Design review of the part built by this model. Coordinates are the model's own, in mm. A direction names the side the tool comes from. Coordinates: 2 decimals unless noted, no trailing zeros. Loops run counter-clockwise (first coordinate to the right, second up) from the corner with the lowest first, then second, coordinate; pieces in that order, holes last. Notation, with made-up numbers: (27.5, 87.25) -> (77.5, 87.25) arc R20 ccw to (77.5, 113.25) -> close; hole circle Ø7 at (-17, 65.5). An arc over 180 degrees is marked (long way). Answer in a Markdown table with one row per item.
Autodesk Fusion 360 part; units mm, degrees
sketch "Sketch1" plane through (0, 0, 0) normal (0, 1, 0) x (1, 0, 0)
  circle A0 centre (0, 0) radius 61
  dimension "d2" = 122
extrude "Extrude1" add sketch "Sketch1" along normal blind 5
sketch "Sketch3" plane through (0, 5, 0) normal (0, 1, 0) x (-1, 0, 0)
  circle A0 centre (0, 0) radius 61
  circle A1 centre (0, 0) radius 61
  circle A2 centre (0, 0) radius 57.25
  dimension "d5" = 114.5
extrude "Extrude2" add sketch "Sketch3" along normal blind 50
sketch "Sketch4" plane through (0, 5, 0) normal (0, 1, 0) x (-1, 0, 0)
  circle A0 centre (0, 0) radius 57.25
  circle A1 centre (0, 0) radius 45
  dimension "d8" = 90
extrude "Extrude3" cut sketch "Sketch4" against normal blind 55 contours A1
(1) To check wall thickness, follow probe 1 along Z at (x, y) = (0, 37); probe 2 along Z at (x, y) = (0, 1). State the ranges of each line that lie inside material, in increasing order.
Evaluation:
| item | result |
|---|---|
| probe 1 | z = -61 to -57.25, 57.25 to 61 |
| probe 2 | z = -61 to -45, 45 to 61 |
(2) Take a section at A-A on z = 29. Give the boundary of the cut face in (x, y), and give its area (3 significant figures).
Evaluation:
| item | result |
|---|---|
| outline | (-53.67, 0) -> (-34.41, 0) -> (-34.41, 5) -> (-49.36, 5) -> (-49.36, 55) -> (-53.67, 55) -> close; (34.41, 0) -> (53.67, 0) -> (53.67, 55) -> (49.36, 55) -> (49.36, 5) -> (34.41, 5) -> close |
| area | 623 mm² |
(3) Tool access review of faces 5 (the flat face through (-5, 0, 45)), 6 (the flat face through (25, 5, 38)): name each direction out of +Z, -Z, +X, -X, +Y, -Y from which nothing blocks a thin tool from reaching the whole face with its end or side.
Evaluation:
| item | result |
|---|---|
| face 5 | +Z, -Z, +X, -X, -Y |
| face 6 | +Y |
(4) Take a section at D-D on z = 50. Give the boundary of the cut face in (x, y), and give its area (3 significant figures).
Evaluation:
| item | result |
|---|---|
| outline | (-34.94, 0) -> (34.94, 0) -> (34.94, 55) -> (27.88, 55) -> (27.88, 5) -> (-27.88, 5) -> (-27.88, 55) -> (-34.94, 55) -> close |
| area | 1,060 mm² |
(5) For pin 1 (5 mm diameter, centred on y = 32, z = 36, fed in from +X); pin 2 (12 mm diameter, centred on y = 22, z = 34.5, fed in from +X); pin 3 (1.5 mm diameter, centred on x = -37, y = 12, fed in from +Z), all flat-tipped, find the tip position at first contact; note any pin that passes through.
Evaluation:
| item | result |
|---|---|
| pin 1 | stops at x = 50.98 |
| pin 2 | stops at x = 53.93 |
| pin 3 | stops at z = 49.06 |
(6) Take a section at C-C on y = 15. Give the boundary of the cut face in (x, z).
Evaluation:
| item | result |
|---|---|
| outline | circle Ø122 at (0, 0); hole circle Ø114.5 at (0, 0) |
(7) Draft analysis for pull direction Z (two halves, no side actions). For faces 1 (the cylindrical face through (12.41, 29.65, 55.89)), 2 (the flat face through (-18, 55, 55)), 3 (the cylindrical face through (-4.021, 27.115, -60.867)), 4 (the cylindrical face through (-20.765, 2.535, -39.923)), state which applies: pulls with the +Z half, pulls with the -Z half, needs draft (parallel to the pull), parting line crosses it, or undercut.
Evaluation:
| item | result |
|---|---|
| face 1 | undercut |
| face 2 | needs draft |
| face 3 | parting line crosses it |
| face 4 | undercut |
